The model under review builds one solid part; all positions refer to its coordinate system, in mm. Face numbers are marked on the shaded views. A direction names the side the tool comes from. Coordinates: 2 decimals unless noted, no trailing zeros. Write each loop counter-clockwise with the first axis right and the second up, starting at its lowest first coordinate (ties: lowest second). Pieces come first, ordered by that corner, then holes.
```python
from build123d import *

# Parameters (mm, degrees)
F1_DEPTH = 50
F3_D     = 6.6
F3_DEPTH = 20
F3_TIP   = 1.9828400428


# Not quite as in the source:
# - a feature names something its author has since deleted; it is built from what else it names


with BuildPart() as f1:
    # F0 (on Top) → F1 (new body)
    with BuildSketch(Plane.XY):
        with BuildLine():
            Line((0, 39), (0, 0))
            Line((0, 0), (17.4234656395, 8.4667937898))
            ThreePointArc((17.4234656395, 8.4667937898), (24, 26), (30.5765343605, 8.4667937898))
            Line((30.5765343605, 8.4667937898), (48, 0))
            Line((48, 0), (48, 39))
            Line((48, 39), (0, 39))
        make_face()
    extrude(amount=F1_DEPTH)

    # F3
    with Locations(Plane(origin=(0, 39, 0), x_dir=(-1, 0, 0), z_dir=(0, 1, 0))):
        with Locations((-41.5, 42.5), (-41.5, 7.5), (-6.5, 7.5), (-6.5, 42.5)):
            Hole(F3_D / 2, depth=F3_DEPTH)
            with Locations((0, 0, -(F3_DEPTH + F3_TIP / 2))):  # 118° drill point
                Cone(0, F3_D / 2, F3_TIP, mode=Mode.SUBTRACT)


solid = f1.part
```
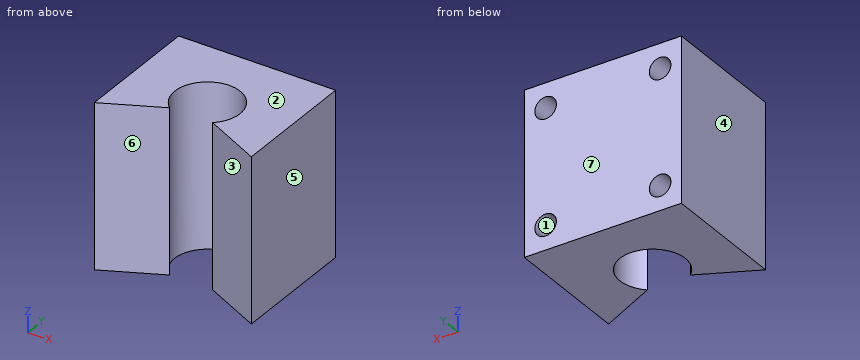
Item 1: Take a section at D-D, the plane y = 16. Write out the cut boundary in (x, z), plus the area to 3 significant figures.
Solved:
outline: (0, 0) - (14, 0) - (14, 50) - (0, 50) - close; (34, 0) - (48, 0) - (48, 50) - (34, 50) - close
area: 1,400 mm2
Item 2: Mouldability with a two-part tool opening along X and no side actions: class the marked faces 4, 5, 6 and 7 as pulls with the +X half, pulls with the -X half, needs draft (parallel to the pull), parting line crosses it, or undercut.
Solved:
face 4: pulls with the -X half
face 5: pulls with the +X half
face 6: undercut
face 7: needs draft
Item 3: For pin 1 (4 mm diameter, centred on x = 22, z = 21.5, fed in from -Y); pin 2 (5.5 mm diameter, centred on x = 41.5, z = 7.5, fed in from +Y); pin 3 (5.5 mm diameter, centred on x = 6.5, z = 42.5, fed in from -Y), all flat-tipped, find the tip position at first contact; note any pin that passes through.
Solved:
pin 1: stops at y = 25.17
pin 2: stops at y = 18.67
pin 3: stops at y = 1.82
Item 4: Take a section at B-B, the plane y = 21. Write out the cut boundary in (x, z), plus the area to 3 significant figures.
Solved:
outline: (0, 0) - (15.34, 0) - (15.34, 50) - (0, 50) - close; (32.66, 0) - (48, 0) - (48, 50) - (32.66, 50) - close; hole circle Ø6.6 at (6.5, 7.5); hole circle Ø6.6 at (6.5, 42.5); hole circle Ø6.6 at (41.5, 7.5); hole circle Ø6.6 at (41.5, 42.5)
area: 1,400 mm2
Item 5: Machinability: for the marked faces 1, 2 and 3, which of the approach directions +Z, -Z, +X, -X, +Y, -Y give a long, thin tool a straight path to every point of the face, cutting with its end or side? Answer none if there is none.
Solved:
face 1: +Y
face 2: +Z, +X, -X, +Y, -Y
face 3: +Z, -Z, -Y
Item 6: Take a section at C-C, the plane x = 32.5. Write out the cut boundary in (y, z), plus the area to 3 significant figures.
Solved:
outline: (7.53, 0) - (10.73, 0) - (10.73, 50) - (7.53, 50) - close; (21.27, 0) - (39, 0) - (39, 50) - (21.27, 50) - close
area: 1,050 mm2
Item 7: To check wall thickness, follow line 1 along Z through (x, y) = (6.5, 31); line 2 along X through (y, z) = (32, 42.5); line 3 along X through (y, z) = (16, 16). State the ranges of each line that lie inside material, in increasing order.
Solved:
line 1: z = 0 to 4.2, 10.8 to 39.2, 45.8 to 50
line 2: x = 0 to 3.2, 9.8 to 38.2, 44.8 to 48
line 3: x = 0 to 14, 34 to 48
Item 8: Take a section at A-A, the plane y = 35. Write out the cut boundary in (x, z), plus the area to 3 significant figures.
Solved:
outline: (0, 0) - (48, 0) - (48, 50) - (0, 50) - close; hole circle Ø6.6 at (6.5, 7.5); hole circle Ø6.6 at (6.5, 42.5); hole circle Ø6.6 at (41.5, 7.5); hole circle Ø6.6 at (41.5, 42.5)
area: 2,260 mm2
